from build123d import *

# Parameters (mm, degrees)
F3_R     = 1.75
F4_DEPTH = 3
F5_R     = 1.75
F6_DEPTH = 3


with BuildPart() as f2:
    # F2: sweep along a path in F1
    with BuildLine(Plane.XY) as f2_path:
        Line((0, -5.9156941882), (30, -5.9156941882))
        ThreePointArc((30, -5.9156941882), (58.2842712475, -17.6314229407), (70, -45.9156941882))
        Line((70, -45.9156941882), (70, -75.9156941882))
    # F0 (on Right) → F2 (sweep)
    with BuildSketch(Plane.YZ):
        with BuildLine():
            Line((-5.9156941882, 10), (1.0843058118, 10))
            Line((1.0843058118, 10), (1.0843058118, -9))
            Line((1.0843058118, -9), (-5.9156941882, -9))
            Line((-5.9156941882, -9), (-5.9156941882, -10.5))
            Line((-5.9156941882, -10.5), (1.0843058118, -10.5))
            ThreePointArc((1.0843058118, -10.5), (3.2056261554, -9.6213203436), (4.0843058118, -7.5))
            Line((4.0843058118, -7.5), (4.0843058118, 8.5))
            ThreePointArc((4.0843058118, 8.5), (3.2056261554, 10.6213203436), (1.0843058118, 11.5))
            Line((1.0843058118, 11.5), (-5.9156941882, 11.5))
            Line((-5.9156941882, 11.5), (-5.9156941882, 10))
        make_face()
    sweep(path=f2_path.line)

    # F3 (on face) → F4 (cut, through all)
    with BuildSketch(Plane.YZ.offset(80)):
        with Locations((-65.9156941882, 0)):
            Circle(F3_R)
    extrude(amount=-F4_DEPTH, mode=Mode.SUBTRACT)

    # F5 (on face) → F6 (cut, through all)
    with BuildSketch(Plane(origin=(0, 4.0843058118, 0), x_dir=(-1, 0, 0), z_dir=(0, 1, 0))):
        with Locations((-10, 0)):
            Circle(F5_R)
    extrude(amount=-F6_DEPTH, mode=Mode.SUBTRACT)


solid = f2.part
For this review, take the finished solid that the model builds, in its own axes (mm). A direction names the side the tool comes from. Round coordinates to 2 decimals unless told otherwise and drop trailing zeros. Order: outer loops, then holes, each group sorted by start corner. A loop starts at its lowest first (then second) coordinate and runs counter-clockwise, first axis right, second up. Notation, with made-up numbers: M -8,-25.5 L 40,-25.5 A19 ccw 40,-4.5 Z; hole C 73.5,-16.5 d4. An arc over 180 degrees is marked long. Write each question's results on one line, items separated by ' | '. Start each with the question number.
1. Add section A-A (z = 0). State the section outline as (x, y) points, then the cut area to 3 significant figures.
2. Draft analysis for pull direction Z (two halves, no side actions). For faces 3 (the face through (79.14, -61.13, 10.6)), 4 (the face through (8.331, 2.605, 0.526)), 5 (the face through (15, 4.084, 0)), state which applies: pulls with the +Z half, pulls with the -Z half, needs draft (parallel to the pull), parting line crosses it, or undercut.
3. To check wall thickness, follow L1, parallel to Z at x = 9.5, y = -3.5; L2, parallel to Y at x = 29, z = -3.25; L3, parallel to X at y = -70.5, z = 3.5. State the ranges of each line that lie inside material, in increasing order. Write a range as [from, to].
4. Add section B-B (x = 10). State the section outline as (y, z) points, then the cut area to 3 significant figures.
5. Add section D-D (y = -70). State the section outline as (x, z) points.
6. Clearance check with flat-ended pins moving along their axes: pin 1 Ø2 at (x, z) = (10, 0) entering from -Y; pin 2 Ø5 at (y, z) = (-29, 8) entering from -X; pin 3 Ø3 at (x, z) = (71, 4) entering from +Y; pin 4 Ø4 at (x, z) = (57.5, -7) entering from +Y. State where each tip first meets the part, or that it passes through.
7. Tool access review of faces 1 (the face through (77, -61, 1)), 2 (the face through (61, -20, -10.5)): name each direction out of +Z, -Z, +X, -X, +Y, -Y from which nothing blocks a thin tool from reaching the whole face with its end or side.
8. Add section C-C (x = 26). State the section outline as (y, z) points, then the cut area to 3 significant figures.
Output values:
1) outline: M 0,1.08 L 8.25,1.08 L 8.25,4.08 L 0,4.08 Z; M 11.75,1.08 L 30,1.08 A47 cw 77,-45.92 L 77,-64.17 L 80,-64.17 L 80,-45.92 A50 ccw 30,4.08 L 11.75,4.08 Z; M 77,-75.92 L 80,-75.92 L 80,-67.67 L 77,-67.67 Z | area: 388 mm^2
2) face 3: pulls with the +Z half | face 4: undercut | face 5: needs draft
3) L1: [-10.5, -9], [10, 11.5] | L2: [1.08, 4.08] | L3: [77, 80]
4) outline: M -5.92,-10.5 L 1.08,-10.5 A3 ccw 4.08,-7.5 L 4.08,-1.75 L 1.08,-1.75 L 1.08,-9 L -5.92,-9 Z; M -5.92,10 L 1.08,10 L 1.08,1.75 L 4.08,1.75 L 4.08,8.5 A3 ccw 1.08,11.5 L -5.92,11.5 Z | area: 72.6 mm^2
5) outline: M 70,-10.5 L 77,-10.5 A3 ccw 80,-7.5 L 80,8.5 A3 ccw 77,11.5 L 70,11.5 L 70,10 L 77,10 L 77,-9 L 70,-9 Z
6) pin 1: through | pin 2: x = 65.51 | pin 3: y = -15.26 | pin 4: y = -2.91
7) face 1: -X, -Y | face 2: -Z, +X, -X, +Y, -Y
8) outline: M -5.92,-10.5 L 1.08,-10.5 A3 ccw 4.08,-7.5 L 4.08,8.5 A3 ccw 1.08,11.5 L -5.92,11.5 L -5.92,10 L 1.08,10 L 1.08,-9 L -5.92,-9 Z | area: 83.1 mm^2
